```python
from build123d import *

# Parameters (mm, degrees)
F0_DEPTH = 1.25
F4_DEPTH = 0.5
F1_DEPTH = 0.625


with BuildPart() as f0:
    # F2 (on Top) → F0 (new body)
    with BuildSketch(Plane.XY):
        with BuildLine():
            ThreePointArc((2.2414386804, -1.2940952255), (2.5, -0.6698729811), (2.588190451, 0))
            ThreePointArc((2.588190451, 0), (2.5, 0.6698729811), (2.2414386804, 1.2940952255))
            ThreePointArc((2.2414386804, 1.2940952255), (1.8301270189, 1.8301270189), (1.2940952255, 2.2414386804))
            ThreePointArc((1.2940952255, 2.2414386804), (0.6698729811, 2.5), (0, 2.588190451))
            ThreePointArc((0, 2.588190451), (-0.6698729811, 2.5), (-1.2940952255, 2.2414386804))
            ThreePointArc((-1.2940952255, 2.2414386804), (-1.8301270189, 1.8301270189), (-2.2414386804, 1.2940952255))
            ThreePointArc((-2.2414386804, 1.2940952255), (-2.5, 0.6698729811), (-2.588190451, 0))
            Line((-2.588190451, 0), (0, 0))
            Line((0, 0), (0, -2.588190451))
            ThreePointArc((0, -2.588190451), (0.6698729811, -2.5), (1.2940952255, -2.2414386804))
            ThreePointArc((1.2940952255, -2.2414386804), (1.8301270189, -1.8301270189), (2.2414386804, -1.2940952255))
        make_face()
        with BuildLine():
            Line((79.283469064, -7.6867534323), (2.588190451, 0))
            ThreePointArc((2.588190451, 0), (2.5, -0.6698729811), (2.2414386804, -1.2940952255))
            Line((2.2414386804, -1.2940952255), (72.5048750257, -32.984810787))
            Line((72.5048750257, -32.984810787), (149.2001536387, -40.6715642193))
            Line((149.2001536387, -40.6715642193), (151.3053811766, -40.5421546968))
            Line((151.3053811766, -40.5421546968), (149.5469054093, -39.3774689938))
            Line((149.5469054093, -39.3774689938), (79.283469064, -7.6867534323))
        make_face()
        with BuildLine():
            ThreePointArc((2.2414386804, 1.2940952255), (2.5, 0.6698729811), (2.588190451, 0))
            Line((2.588190451, 0), (79.283469064, 7.6867534323))
            Line((79.283469064, 7.6867534323), (149.5469054093, 39.3774689938))
            Line((149.5469054093, 39.3774689938), (151.3053811766, 40.5421546968))
            Line((151.3053811766, 40.5421546968), (149.2001536387, 40.6715642193))
            Line((149.2001536387, 40.6715642193), (72.5048750257, 32.984810787))
            Line((72.5048750257, 32.984810787), (2.2414386804, 1.2940952255))
        make_face()
        with BuildLine():
            ThreePointArc((1.2940952255, 2.2414386804), (1.8301270189, 1.8301270189), (2.2414386804, 1.2940952255))
            Line((2.2414386804, 1.2940952255), (64.8181215934, 46.298658277))
            Line((64.8181215934, 46.298658277), (109.8226846449, 108.87534119))
            Line((109.8226846449, 108.87534119), (110.7632264798, 110.7632264798))
            Line((110.7632264798, 110.7632264798), (108.87534119, 109.8226846449))
            Line((108.87534119, 109.8226846449), (46.298658277, 64.8181215934))
            Line((46.298658277, 64.8181215934), (1.2940952255, 2.2414386804))
        make_face()
        with BuildLine():
            Line((64.8181215934, -46.298658277), (2.2414386804, -1.2940952255))
            ThreePointArc((2.2414386804, -1.2940952255), (1.8301270189, -1.8301270189), (1.2940952255, -2.2414386804))
            Line((1.2940952255, -2.2414386804), (46.298658277, -64.8181215934))
            Line((46.298658277, -64.8181215934), (108.87534119, -109.8226846449))
            Line((108.87534119, -109.8226846449), (110.7632264798, -110.7632264798))
            Line((110.7632264798, -110.7632264798), (109.8226846449, -108.87534119))
            Line((109.8226846449, -108.87534119), (64.8181215934, -46.298658277))
        make_face()
        with BuildLine():
            ThreePointArc((0, 2.588190451), (0.6698729811, 2.5), (1.2940952255, 2.2414386804))
            Line((1.2940952255, 2.2414386804), (32.984810787, 72.5048750257))
            Line((32.984810787, 72.5048750257), (40.6715642193, 149.2001536387))
            Line((40.6715642193, 149.2001536387), (40.5421546968, 151.3053811766))
            Line((40.5421546968, 151.3053811766), (39.3774689938, 149.5469054093))
            Line((39.3774689938, 149.5469054093), (7.6867534323, 79.283469064))
            Line((7.6867534323, 79.283469064), (0, 2.588190451))
        make_face()
        with BuildLine():
            Line((32.984810787, -72.5048750257), (1.2940952255, -2.2414386804))
            ThreePointArc((1.2940952255, -2.2414386804), (0.6698729811, -2.5), (0, -2.588190451))
            Line((0, -2.588190451), (7.6867534323, -79.283469064))
            Line((7.6867534323, -79.283469064), (39.3774689938, -149.5469054093))
            Line((39.3774689938, -149.5469054093), (40.5421546968, -151.3053811766))
            Line((40.5421546968, -151.3053811766), (40.6715642193, -149.2001536387))
            Line((40.6715642193, -149.2001536387), (32.984810787, -72.5048750257))
        make_face()
        with BuildLine():
            ThreePointArc((-1.2940952255, 2.2414386804), (-0.6698729811, 2.5), (0, 2.588190451))
            Line((0, 2.588190451), (-7.6867534323, 79.283469064))
            Line((-7.6867534323, 79.283469064), (-39.3774689938, 149.5469054093))
            Line((-39.3774689938, 149.5469054093), (-40.5421546968, 151.3053811766))
            Line((-40.5421546968, 151.3053811766), (-40.6715642193, 149.2001536387))
            Line((-40.6715642193, 149.2001536387), (-32.984810787, 72.5048750257))
            Line((-32.984810787, 72.5048750257), (-1.2940952255, 2.2414386804))
        make_face()
        with BuildLine():
            Line((-7.6867534323, -79.283469064), (0, -2.588190451))
            ThreePointArc((0, -2.588190451), (-0.6698729811, -2.5), (-1.2940952255, -2.2414386804))
            Line((-1.2940952255, -2.2414386804), (-32.984810787, -72.5048750257))
            Line((-32.984810787, -72.5048750257), (-40.6715642193, -149.2001536387))
            Line((-40.6715642193, -149.2001536387), (-40.5421546968, -151.3053811766))
            Line((-40.5421546968, -151.3053811766), (-39.3774689938, -149.5469054093))
            Line((-39.3774689938, -149.5469054093), (-7.6867534323, -79.283469064))
        make_face()
        Polygon((-1.2940952255, -2.2414386804), (0, -2.588190451), (0, 0), align=None)
        with BuildLine():
            ThreePointArc((-1.2940952255, -2.2414386804), (-0.6698729811, -2.5), (0, -2.588190451))
            Line((0, -2.588190451), (-1.2940952255, -2.2414386804))
        make_face()
        with BuildLine():
            ThreePointArc((-2.2414386804, 1.2940952255), (-1.8301270189, 1.8301270189), (-1.2940952255, 2.2414386804))
            Line((-1.2940952255, 2.2414386804), (-46.298658277, 64.8181215934))
            Line((-46.298658277, 64.8181215934), (-108.87534119, 109.8226846449))
            Line((-108.87534119, 109.8226846449), (-110.7632264798, 110.7632264798))
            Line((-110.7632264798, 110.7632264798), (-109.8226846449, 108.87534119))
            Line((-109.8226846449, 108.87534119), (-64.8181215934, 46.298658277))
            Line((-64.8181215934, 46.298658277), (-2.2414386804, 1.2940952255))
        make_face()
        with BuildLine():
            Line((-46.298658277, -64.8181215934), (-1.2940952255, -2.2414386804))
            ThreePointArc((-1.2940952255, -2.2414386804), (-1.8301270189, -1.8301270189), (-2.2414386804, -1.2940952255))
            Line((-2.2414386804, -1.2940952255), (-64.8181215934, -46.298658277))
            Line((-64.8181215934, -46.298658277), (-109.8226846449, -108.87534119))
            Line((-109.8226846449, -108.87534119), (-110.7632264798, -110.7632264798))
            Line((-110.7632264798, -110.7632264798), (-108.87534119, -109.8226846449))
            Line((-108.87534119, -109.8226846449), (-46.298658277, -64.8181215934))
        make_face()
        Polygon((-2.2414386804, -1.2940952255), (-1.2940952255, -2.2414386804), (0, 0), align=None)
        with BuildLine():
            ThreePointArc((-2.2414386804, -1.2940952255), (-1.8301270189, -1.8301270189), (-1.2940952255, -2.2414386804))
            Line((-1.2940952255, -2.2414386804), (-2.2414386804, -1.2940952255))
        make_face()
        Polygon((-2.2414386804, -1.2940952255), (0, 0), (-2.588190451, 0), align=None)
        with BuildLine():
            ThreePointArc((-2.588190451, 0), (-2.5, 0.6698729811), (-2.2414386804, 1.2940952255))
            Line((-2.2414386804, 1.2940952255), (-72.5048750257, 32.984810787))
            Line((-72.5048750257, 32.984810787), (-149.2001536387, 40.6715642193))
            Line((-149.2001536387, 40.6715642193), (-151.3053811766, 40.5421546968))
            Line((-151.3053811766, 40.5421546968), (-149.5469054093, 39.3774689938))
            Line((-149.5469054093, 39.3774689938), (-79.283469064, 7.6867534323))
            Line((-79.283469064, 7.6867534323), (-2.588190451, 0))
        make_face()
        with BuildLine():
            Line((-72.5048750257, -32.984810787), (-2.2414386804, -1.2940952255))
            ThreePointArc((-2.2414386804, -1.2940952255), (-2.5, -0.6698729811), (-2.588190451, 0))
            Line((-2.588190451, 0), (-79.283469064, -7.6867534323))
            Line((-79.283469064, -7.6867534323), (-149.5469054093, -39.3774689938))
            Line((-149.5469054093, -39.3774689938), (-151.3053811766, -40.5421546968))
            Line((-151.3053811766, -40.5421546968), (-149.2001536387, -40.6715642193))
            Line((-149.2001536387, -40.6715642193), (-72.5048750257, -32.984810787))
        make_face()
        with BuildLine():
            ThreePointArc((-2.588190451, 0), (-2.5, -0.6698729811), (-2.2414386804, -1.2940952255))
            Line((-2.2414386804, -1.2940952255), (-2.588190451, 0))
        make_face()
    extrude(amount=F0_DEPTH)

    # F3 (on face) → F4 (join)
    with BuildSketch(Plane.XY):
        with BuildLine():
            ThreePointArc((-40.6715642193, -149.2001536387), (-42.407285452, -153.4761541969), (-38.1479036577, -151.7000416718))
            ThreePointArc((-38.1479036577, -151.7000416718), (-38.4769491833, -150.4603011061), (-39.3774689938, -149.5469054093))
            Line((-39.3774689938, -149.5469054093), (-40.5421546968, -151.3053811766))
            Line((-40.5421546968, -151.3053811766), (-40.6715642193, -149.2001536387))
        make_face()
        with BuildLine():
            Line((-40.5421546968, -151.3053811766), (-39.3774689938, -149.5469054093))
            ThreePointArc((-39.3774689938, -149.5469054093), (-40.000856045, -149.2852271061), (-40.6715642193, -149.2001536387))
            Line((-40.6715642193, -149.2001536387), (-40.5421546968, -151.3053811766))
        make_face()
    extrude(amount=F4_DEPTH)

    # F5 (on face) → F1 (cut)
    with BuildSketch(Plane(origin=(0, 0, 0), x_dir=(1, 0, 0), z_dir=(0, 0, -1))):
        Polygon((40.6715642193, 149.2001536387), (40.5421546968, 151.3053811766), (39.3774689938, 149.5469054093), align=None)
        Polygon((109.8226846449, 108.87534119), (110.7632264798, 110.7632264798), (108.87534119, 109.8226846449), align=None)
        Polygon((151.3053811766, 40.5421546968), (149.2001536387, 40.6715642193), (149.5469054093, 39.3774689938), align=None)
        Polygon((149.5469054093, -39.3774689938), (149.2001536387, -40.6715642193), (151.3053811766, -40.5421546968), align=None)
        Polygon((109.8226846449, -108.87534119), (108.87534119, -109.8226846449), (110.7632264798, -110.7632264798), align=None)
        Polygon((40.5421546968, -151.3053811766), (40.6715642193, -149.2001536387), (39.3774689938, -149.5469054093), align=None)
        Polygon((-40.5421546968, -151.3053811766), (-39.3774689938, -149.5469054093), (-40.6715642193, -149.2001536387), align=None)
        Polygon((-109.8226846449, -108.87534119), (-110.7632264798, -110.7632264798), (-108.87534119, -109.8226846449), align=None)
        Polygon((-149.2001536387, -40.6715642193), (-149.5469054093, -39.3774689938), (-151.3053811766, -40.5421546968), align=None)
        Polygon((-149.5469054093, 39.3774689938), (-149.2001536387, 40.6715642193), (-151.3053811766, 40.5421546968), align=None)
        Polygon((-109.8226846449, 108.87534119), (-108.87534119, 109.8226846449), (-110.7632264798, 110.7632264798), align=None)
    extrude(amount=-F1_DEPTH, mode=Mode.SUBTRACT)


solid = f0.part
```
Work out the finished part from the listing and answer in its coordinate system (mm). A direction names the side the tool comes from. Coordinates: 2 decimals unless noted, no trailing zeros. Write each loop counter-clockwise with the first axis right and the second up, starting at its lowest first coordinate (ties: lowest second). Pieces come first, ordered by that corner, then holes. Notation, with made-up numbers: (64, 66.25) - (86, 66.25) arc R11 ccw to (86, 80.25) - close; hole circle Ø3 at (32.25, 80). An arc over 180 degrees is marked (long way). Answer as a JSON object with one key per item and string values.
Q1. Which of the six approach directions +Z, -Z, +X, -X, +Y, -Y give full straight-line access (tool end or side, diameter ignored) to faces 4 (the flat face through (77.149, -87.005, 0.616)), 5 (the flat face through (-36.774, -110.316, 0.616)), 6 (the flat face through (-23.3, 113.9, 0.6))?
Results list:
{"face 4": "+Z, -Z, -Y", "face 5": "+Z, -Z", "face 6": "+Z, -Z, +Y"}
Q2. Find section B-B (y = 28). Write down the section's boundary in (x, z), plus the area to 3 significant figures.
Results list:
{"outline": "(-124.32, 0) - (-61.45, 0) - (-61.45, 1.25) - (-124.32, 1.25) - close; (-39.37, 0) - (-19.82, 0) - (-19.82, 1.25) - (-39.37, 1.25) - close; (-12.91, 0) - (-2.55, 0) - (-2.55, 1.25) - (-12.91, 1.25) - close; (2.55, 0) - (12.91, 0) - (12.91, 1.25) - (2.55, 1.25) - close; (19.82, 0) - (39.37, 0) - (39.37, 1.25) - (19.82, 1.25) - close; (61.45, 0) - (124.32, 0) - (124.32, 1.25) - (61.45, 1.25) - close", "area": "232 mm^2"}
Q3. Consider L1, parallel to X at y = -107.5, z = 1; L2, parallel to Y at x = -86, z = 0.25; L3, parallel to Y at x = 109, z = 0.8. Determine where each line is inside the solid, lowest interval first. Write a range as from..to.
Results list:
{"L1": "x = -108.83..-105.65, -36.49..-20.41, 20.41..36.49, 105.65..108.83", "L2": "y = -93.37..-75.75, -34.34..-10.72, 10.72..34.34, 75.75..93.37", "L3": "y = -109.88..-107.73, -36.64..-21.09, 21.09..36.64, 107.73..109.88"}
Q4. Given pin 1 Ø0.9 at (x, y) = (110, 110) entering from -Z (3 decimals), flat-ended and moving along its own axis, determine where the tip first touches the part or whether it passes through.
Results list:
{"pin 1": "stops at z = 0.625"}
Q5. Find section A-A (x = 119.5). Write down the section's boundary in (y, z), plus the area to 3 significant figures.
Results list:
{"outline": "(-37.69, 0) - (-25.83, 0) - (-25.83, 1.25) - (-37.69, 1.25) - close; (25.83, 0) - (37.69, 0) - (37.69, 1.25) - (25.83, 1.25) - close", "area": "29.7 mm^2"}
Q6. For a pull along X with two mould halves and no side action, classify faces 1 (the flat face through (33.968, -24.111, 0.616)), 2 (the flat face through (113.9, 23.3, 0.6)), 3 (the flat face through (-1, -2, 0)) as pulls with the +X half, pulls with the -X half, needs draft (parallel to the pull), parting line crosses it, or undercut.
Results list:
{"face 1": "undercut", "face 2": "pulls with the +X half", "face 3": "needs draft"}
Q7. Find section C-C (x = 24). Write down the section's boundary in (y, z), plus the area to 3 significant figures.
Results list:
{"outline": "(-115.45, 0) - (-52.58, 0) - (-52.58, 1.25) - (-115.45, 1.25) - close; (-33.81, 0) - (-16.94, 0) - (-16.94, 1.25) - (-33.81, 1.25) - close; (-11.11, 0) - (-2.15, 0) - (-2.15, 1.25) - (-11.11, 1.25) - close; (2.15, 0) - (11.11, 0) - (11.11, 1.25) - (2.15, 1.25) - close; (16.94, 0) - (33.81, 0) - (33.81, 1.25) - (16.94, 1.25) - close; (52.58, 0) - (115.45, 0) - (115.45, 1.25) - (52.58, 1.25) - close", "area": "222 mm^2"}
Q8. Find section D-D (x = -51). Write down the section's boundary in (y, z).
Results list:
{"outline": "(-68.2, 0) - (-36.36, 0) - (-36.36, 1.25) - (-68.2, 1.25) - close; (-23.29, 0) - (-4.85, 0) - (-4.85, 1.25) - (-23.29, 1.25) - close; (4.85, 0) - (23.29, 0) - (23.29, 1.25) - (4.85, 1.25) - close; (36.36, 0) - (68.2, 0) - (68.2, 1.25) - (36.36, 1.25) - close"}
